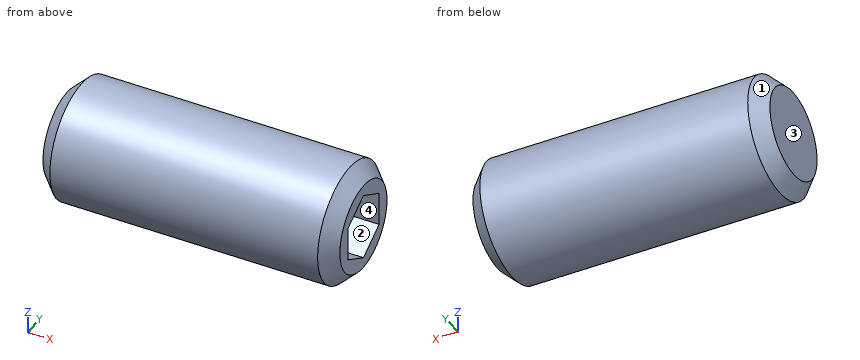
Autodesk Inventor part; units mm, degrees
ref_plane "Work Plane1" through (7.9375, 0, 0) normal (0, 0.5, 0.866) x (1, 0, 0)
ref_plane "YZ Plane" through (0, 0, 0) normal (1, 0, 0) x (0, 1, 0)
ref_plane "XZ Plane" through (0, 0, 0) normal (0, 1, 0) x (-1, 0, 0)
sketch "Sketch1" plane through (0, 0, 0) normal (0, 0, 1) x (1, 0, 0)
  line L0 (0, 0) -> (11.6417, 0)
  line L1 (15.875, 1.8331) -> (15.875, 3.175)
  line L2 (15.875, 3.175) -> (0, 3.175)
  line L3 (15.875, 1.8331) -> (12.7, 1.8331)
  line L4 (12.7, 1.8331) -> (11.6417, 0)
  line L5 (0, -0.635) -> (0, 3.81)
  line L6 (0, 3.175) -> (0, 0)
  dimension "d0" = 3.175
  dimension "d1" = 60
  dimension "d2" = 6.35
  dimension "d3" = 3.6662
  dimension "d5" = 15.875
revolve "Body" add sketch "Sketch1" angle 360 about axis through (0, 0, 0) along (1, 0, 0)
chamfer "Chamfer1" distance 0.7791 angle 45 1 edges at (15.875, -3.175, 0) measured on face at (15.875, 2.6792, -0.3995)
sketch "Sketch2" plane through (15.875, 0, 0) normal (1, 0, 0) x (0, 0, -1)
  circle A0 centre (0, 0) radius 1.8331
  line L0 (-0.9165, 1.5875) -> (0.9165, 1.5875)
  line L1 (0.9165, 1.5875) -> (1.8331, 0)
  line L2 (1.8331, 0) -> (0.9165, -1.5875)
  line L3 (0.9165, -1.5875) -> (-0.9165, -1.5875)
  line L4 (-0.9165, -1.5875) -> (-1.8331, 0)
  line L5 (-1.8331, 0) -> (-0.9165, 1.5875)
  point P0 (0, 0)
  point P1 (0, 0)
extrude "Slot" add sketch "Sketch2" against normal up to next contours L1 A0 | A0 L2 | L0 A0 | A0 L3 | L5 A0 | A0 L4
thread "Thread"
chamfer "Chamfer2" distance 0.7791 angle 45 1 edges at (0, -3.175, 0) measured on face at (5.032, 3.1647, -0.2555)
ref_plane "Work Plane1" through (7.9375, 0, 0) normal (0, 0.5, 0.866) x (1, 0, 0)
equation "\"d7\" = -0.5 * GD1 + 0.5 * NND"
equation "\"d8\" = FAWI"
equation "\"d29\" = -0.5 * GD1 + 0.5 * NND"
equation "\"d11\" = NLG"
equation "\"d13\" = -0.5 * GD1 + 0.5 * NND"
equation "\"d14\" = FAWI"
equation "\"d30\" = -0.5 * GD1 + 0.5 * NND"
equation "\"d0\" = INTI"
equation "\"d2\" = NND"
equation "\"d3\" = 1.1547 * SW"
equation "\"d5\" = NLG"
equation "\"NND\" = 6.35"
equation "\"NLG\" = 15.875"
equation "\"INTI\" = 3.175"
equation "\"FAWI\" = 45deg"
equation "\"SW\" = 3.175"
equation "\"GD1\" = 4.79189"
equation "\"FAWI1\" = 45deg"
equation "\"SPD\" = 3.3528"
equation "\"SEWI\" = 90deg"
equation "\"TOA\" = 30deg"
equation "\"ZLG\" = 1.7018"
equation "\"ZD\" = 3.9624"
equation "\"HHPTC\" = 1.27"
equation "\"THREADDIA\" = 6.35"
equation "\"OPR\" = 4.7752"
equation "\"E0\" = 1.155 * SW"
properties part number "ANSI B18.3 - 1/4-20 UNC x 0.625" material "Steel, Mild"
Could you check a few things on this model? Use its own coordinates, in mm. Face numbers are marked on the shaded views. Coordinates: 2 decimals unless noted, no trailing zeros. Write each loop counter-clockwise with the first axis right and the second up, starting at its lowest first coordinate (ties: lowest second). Pieces come first, ordered by that corner, then holes. Notation, with made-up numbers: (55.25, -12) - (82.25, -12) arc R32 ccw to (82.25, 22) - close; hole circle Ø4 at (-24.5, -12). An arc over 180 degrees is marked (long way). Write item = value, one per line.
1) We'd pull the mould along Z, two halves only. Please class the marked faces 1, 2, 3 and 4: +Z half, -Z half, draft (parallel to the pull), parting line (faces both ways), or undercut.
Result set:
face_1 = parting line
face_2 = undercut
face_3 = draft
face_4 = undercut
2) Suppose I cut it at A-A on x = 5.25. Please give me the cut outline in (y, z) (3 decimals), plus the area to 3 significant figures.
Result set:
outline = circle Ø6.35 at (0, 0)
area = 31.7 mm2
3) Suppose I cut it at B-B on x = 12.25. Please give me the cut outline in (y, z) (3 decimals), plus the area to 3 significant figures.
Result set:
outline = circle Ø6.35 at (0, 0); hole circle Ø2.107 at (0, 0)
area = 28.2 mm2
4) Please list where these lines run through material, in increasing order: line 1 (Y direction, x = 13, z = 1.75); line 2 (Z direction, x = 12.75, y = 1.25); line 3 (Y direction, x = 14.5, z = -2.75). Write a range as [from, to].
Result set:
line_1 = [-2.65, -0.14], [0.14, 2.65]
line_2 = [-2.92, -1.11], [1.11, 2.92]
line_3 = [-1.59, 1.59]
5) Will these pins go through, and if not, where does the flat tip stop? pin 1 Ø1.5 at (x, y) = (7, 1.5) entering from +Z; pin 2 Ø2 at (x, z) = (7, 1.5) entering from -Y.
Result set:
pin_1 = 3.09
pin_2 = -3.14
